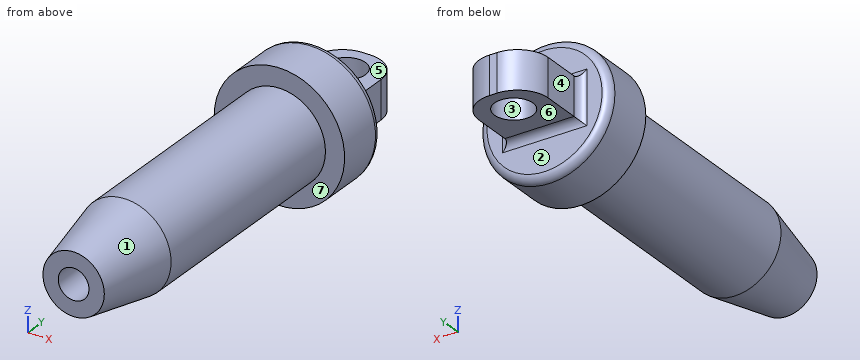
Autodesk Inventor part; units mm, degrees
ref_plane "YZ Plane" through (0, 0, 0) normal (1, 0, 0) x (0, 1, 0)
ref_plane "XZ Plane" through (0, 0, 0) normal (0, 1, 0) x (-1, 0, 0)
ref_plane "XY Plane" through (0, 0, 0) normal (0, 0, 1) x (1, 0, 0)
sketch "Szkic1" plane through (0, 0, 0) normal (0, 1, 0) x (-1, 0, 0)
  circle A0 centre (0, 0) radius 8.5
  dimension "d0" = 17
extrude "Wyciągnięcie proste1" add sketch "Szkic1" along normal blind 7
sketch "Szkic2" plane through (0, 7, 0) normal (0, 1, 0) x (1, 0, 0)
  line L0 (4.5, -2.5) -> (-4.5, -2.5)
  line L1 (-4.5, -2.5) -> (-4.5, 2.5)
  line L2 (-4.5, 2.5) -> (4.5, 2.5)
  line L3 (4.5, 2.5) -> (4.5, -2.5)
  line L4 (4.5, -2.5) -> (-4.5, 2.5) construction
  line L5 (-4.5, -2.5) -> (4.5, 2.5) construction
  point P0 (0, 0)
  dimension "d3" = 9
  dimension "d4" = 5
extrude "Wyciągnięcie proste2" add sketch "Szkic2" along normal blind 10
fillet "Zaokrąglenie1" radius 4 2 edges at (4.5, 17, 0) (-4.5, 17, 0)
sketch "Szkic3" plane through (-4.5, 7, 2.5) normal (0, 0, 1) x (1, 0, 0)
  arc A0 (9, 6) -> (5, 10) centre (5, 6) ccw
  arc A1 (4, 10) -> (0, 6) centre (4, 6) ccw
  circle A2 centre (4.5, 6) radius 2.5
  point P0 (4.5, -7)
  dimension "d8" = 5
extrude "Wyciągnięcie proste3" cut sketch "Szkic3" against normal blind 10
fillet "Zaokrąglenie2" radius 1 1 edges at (8.5, 7, 0)
fillet "Zaokrąglenie3" radius 1 4 edges at (0, 7, 2.5) (4.5, 7, 0) (0, 7, -2.5) (-4.5, 7, 0)
sketch "Szkic4" plane through (0, 0, 0) normal (0, -1, 0) x (1, 0, 0)
  circle A0 centre (0, 0) radius 6
  circle A1 centre (0, 0) radius 4.5
  dimension "d13" = 12
  dimension "d21" = 9
extrude "Wyciągnięcie proste4" add sketch "Szkic4" along normal blind 30 from surface at 0
thread "Gwint1"
sketch "Szkic5" plane through (0, -30, 0) normal (0, -1, 0) x (1, 0, 0)
  circle A0 centre (0, 0) radius 2
  circle A1 centre (0, 0) radius 6
  dimension "d22" = 4
extrude "Wyciągnięcie proste5" add sketch "Szkic5" along normal blind 10
chamfer "Faza2" distance 2 distance2 10 1 edges at (-6, -40, 0) measured on face at (4.5892, -40, -0.6382)
properties part number "Korpus" material "Aluminum 6061"
The listing builds one solid part. Answer for the finished solid, in the listing's coordinates (mm). Face numbers are marked on the shaded views. A direction names the side the tool comes from. Round coordinates to 2 decimals unless told otherwise and drop trailing zeros. Loops run counter-clockwise (first coordinate to the right, second up) from the corner with the lowest first, then second, coordinate; pieces in that order, holes last. Notation, with made-up numbers: (20, -33) - (48, -33) arc R32 cw to (48, 0) - close; hole circle Ø4 at (-0.5, 67). An arc over 180 degrees is marked (long way). Use one line per item in the form item = value. Start each with the question number.
1. Consider line 1 (Y direction, x = 0, z = 1); line 2 (Y direction, x = 1.25, z = 3.5); line 3 (X direction, y = -33, z = -0.75). Determine where each line is inside the solid, lowest interval first. Write a range as [from, to].
2. A tool of negligible diameter and unlimited length cuts with its end or side. For the marked faces 5, 6 and 7, from which of +Z, -Z, +X, -X, +Y, -Y can it reach the whole face along a straight path? Write none if from no direction.
3. For a pull along Y with two mould halves and no side action, classify the marked faces 1, 2, 3 and 4 as pulls with the +Y half, pulls with the -Y half, needs draft (parallel to the pull), parting line crosses it, or undercut.
4. The part is cut by section D-D on y = 2.5. Determine the outline of the cut face in (x, z).
5. The part is cut by section C-C on y = -19.5. Determine the outline of the cut face in (x, z).
6. Given pin 1 Ø10 at (x, z) = (-4.5, -6.5) entering from +Y; pin 2 Ø1 at (x, z) = (1, 0.5) entering from -Y; pin 3 Ø5 at (x, y) = (3, -28.5) entering from -Z, each flat-ended and moving along its own axis, determine where each tip first touches the part or whether it passes through.
Geometry check:
q1.line_1 = [0, 10.5], [15.5, 17]
q1.line_2 = [-40, -30], [0, 7]
q1.line_3 = [-5.35, -1.85], [1.85, 5.35]
q2.face_5 = +Z, +X, -X, +Y
q2.face_6 = -Z, +X, -X, +Y
q2.face_7 = -Y
q3.face_1 = pulls with the -Y half
q3.face_2 = pulls with the +Y half
q3.face_3 = undercut
q3.face_4 = needs draft
q4.outline = circle Ø17 at (0, 0)
q5.outline = circle Ø12 at (0, 0); hole circle Ø9 at (0, 0)
q6.pin_1 = 16.87
q6.pin_2 = 0
q6.pin_3 = -5.98
